```python
from build123d import *

# Parameters (mm, degrees)
BOSS_EXTRUDE1_DEPTH        = 320.675
BOSS_EXTRUDE1_DEPTH_BACK   = 320.675
SKETCH3_W                  = 50.8
SKETCH3_H                  = 25.4
SKETCH3_W_2                = 44.45
SKETCH3_H_2                = 19.05
CUT_EXTRUDE1_DEPTH         = 323.680609311
CUT_EXTRUDE1_DEPTH_BACK    = 323.680609311
SKETCH8_R                  = 14.2875
CUT_EXTRUDE2_DEPTH         = 323.680609311
F_10_CLEARANCE_HOLE1_D     = 4.9784
F_10_CLEARANCE_HOLE1_DEPTH = 5.08
F_10_CLEARANCE_HOLE1_TIP   = 1.495662253
F_10_CLEARANCE_HOLE2_D     = 4.9784
F_10_CLEARANCE_HOLE3_D     = 4.9784
F_10_CLEARANCE_HOLE3_DEPTH = 3.302
F_10_CLEARANCE_HOLE3_TIP   = 1.495662253


with BuildPart() as part:
    # Sketch3 → Boss-Extrude1 (new, two sides: drawn at the far end of the back side and taken through both)
    with BuildSketch(Plane.XY.offset(-BOSS_EXTRUDE1_DEPTH_BACK)):
        Rectangle(SKETCH3_W, SKETCH3_H)
        Rectangle(SKETCH3_W_2, SKETCH3_H_2, mode=Mode.SUBTRACT)
    extrude(amount=BOSS_EXTRUDE1_DEPTH + BOSS_EXTRUDE1_DEPTH_BACK)

    # Sketch4 → Cut-Extrude1 (cut, two sides: drawn at the far end of the back side and taken through both)
    with BuildSketch(Plane(origin=(0, 12.7, 0), x_dir=(1, 0, 0), z_dir=(0, 1, 0)).offset(-CUT_EXTRUDE1_DEPTH_BACK)):
        Polygon((1322.117470931, -320.675), (25.4, -320.675), (-25.4, -320.675), (25.4, -305.627354456), (1268.718301677, 62.660305034), (3837.350959621, 420.474595165), (3890.750128875, 37.139290131), align=None)
    extrude(amount=CUT_EXTRUDE1_DEPTH + CUT_EXTRUDE1_DEPTH_BACK, mode=Mode.SUBTRACT)

    # Sketch8 → Cut-Extrude2 (cut, through all)
    with BuildSketch(Plane(origin=(0, 12.7, 0), x_dir=(1, 0, 0), z_dir=(0, 1, 0))):
        with Locations(Location((0, 266.954, 0), (0, 0, 180))):
            Circle(SKETCH8_R)
    extrude(amount=-CUT_EXTRUDE2_DEPTH, mode=Mode.SUBTRACT)

    # #10 Clearance Hole1
    with Locations(Plane(origin=(0, 12.7, 0), x_dir=(1, 0, 0), z_dir=(0, 1, 0))):
        with Locations((-12.7762, -284.753033923), (12.6238, -284.753033923), (12.6238, -301.263033923), (-12.7762, -301.263033923)):
            Hole(F_10_CLEARANCE_HOLE1_D / 2, depth=F_10_CLEARANCE_HOLE1_DEPTH)
            with Locations((0, 0, -(F_10_CLEARANCE_HOLE1_DEPTH + F_10_CLEARANCE_HOLE1_TIP / 2))):  # 118° drill point
                Cone(0, F_10_CLEARANCE_HOLE1_D / 2, F_10_CLEARANCE_HOLE1_TIP, mode=Mode.SUBTRACT)

    # #10 Clearance Hole2 (through all)
    with Locations(Plane(origin=(25.4, 0, 0), x_dir=(0, 0, -1), z_dir=(1, 0, 0))):
        with Locations((-282.536770585, -6.148316496), (-263.486770585, -6.148316496), (-238.125, -6.148316496), (3.175, -6.35), (28.575, -6.35), (53.975, -6.35), (79.375, -6.35), (104.775, -6.35)):
            Hole(F_10_CLEARANCE_HOLE2_D / 2)

    # #10 Clearance Hole3
    with Locations(Plane(origin=(25.4, 0, 0), x_dir=(0, 0, -1), z_dir=(1, 0, 0))):
        with Locations((269.673316496, -6.388229415), (295.073316496, -6.388229415), (314.123316496, -6.388229415)):
            Hole(F_10_CLEARANCE_HOLE3_D / 2, depth=F_10_CLEARANCE_HOLE3_DEPTH)
            with Locations((0, 0, -(F_10_CLEARANCE_HOLE3_DEPTH + F_10_CLEARANCE_HOLE3_TIP / 2))):  # 118° drill point
                Cone(0, F_10_CLEARANCE_HOLE3_D / 2, F_10_CLEARANCE_HOLE3_TIP, mode=Mode.SUBTRACT)


solid = part.part
```
The listing builds one solid part. Answer for the finished solid, in the listing's coordinates (mm). A direction names the side the tool comes from. Round coordinates to 2 decimals unless told otherwise and drop trailing zeros. Order: outer loops, then holes, each group sorted by start corner. A loop starts at its lowest first (then second) coordinate and runs counter-clockwise, first axis right, second up. Notation, with made-up numbers: (-5.5, 32.25) - (52.5, 32.25) arc R15 cw to (52.5, 47.25) - close; hole circle Ø4 at (15.5, 79). An arc over 180 degrees is marked (long way). Put each result on its own line as item: value. Start each with the question number.
(1) For faces 1 (the flat face through (0, -9.525, -5)), 2 (the flat face through (-25.4, 0, -4)), determine the directions among +Z, -Z, +X, -X, +Y, -Y from which every point of the face is accessible in a straight line to the end or side of a thin tool.
(2) Find section B-B (z = -239). Give the vertices of the cut face in (x, y) (3 decimals), plus the area to 3 significant figures.
(3) Find section C-C (x = 0). Give the vertices of the cut face in (y, z) (1 decimal), plus the area to 3 significant figures.
(4) Determine the mould class of faces 3 (the flat face through (0, 12.7, -4)), 4 (the flat face through (0, 9.525, -5)), 5 (the cylindrical face through (-6.59, -11.09, -279.63)) for opening direction Y: released by +Y, released by -Y, zero draft, split by the parting line, or undercut.
(5) Find section A-A (y = 2.75). Give the vertices of the cut face in (x, z) (3 decimals).
(6) Straight lines are drawn through the part: probe 1 along Y at (x, z) = (-8.5, 202.5) (3 decimals); probe 2 along X at (y, z) = (8.25, -47) (3 decimals); probe 3 along Y at (x, z) = (23.5, -1). For each, find the intervals that lie inside material, in ascending order. Write a range as from..to.
Reply:
1. face 1: +Z, -Z
1. face 2: +Z, -Z, -X, +Y, -Y
2. outline: (-25.4, -12.7) - (25.4, -12.7) - (25.4, 12.7) - (-25.4, 12.7) - close; hole (-22.225, -9.525) - (22.225, -9.525) - (22.225, 9.525) - (-22.225, 9.525) - close
2. area: 444 mm^2
3. outline: (-12.7, -320.7) - (-9.5, -320.7) - (-9.5, -281.2) - (-12.7, -281.2) - close; (-12.7, -252.7) - (-9.5, -252.7) - (-9.5, 313.2) - (-12.7, 313.2) - close; (9.5, -320.7) - (12.7, -320.7) - (12.7, -281.2) - (9.5, -281.2) - close; (9.5, -252.7) - (12.7, -252.7) - (12.7, 313.2) - (9.5, 313.2) - close
3. area: 3,840 mm^2
4. face 3: released by +Y
4. face 4: undercut
4. face 5: zero draft
5. outline: (-25.4, -320.675) - (-22.225, -320.675) - (-22.225, 319.735) - (-25.4, 320.675) - close; (22.225, -320.675) - (25.4, -320.675) - (25.4, 305.627) - (22.225, 306.568) - close
6. probe 1: -12.7..-9.525, 9.525..12.7
6. probe 2: -25.4..-22.225, 22.225..25.4
6. probe 3: -12.7..-7.56, -5.14..12.7
